The listing builds one solid part. Answer for the finished solid, in the listing's coordinates (mm). A direction names the side the tool comes from. Coordinates: 2 decimals unless noted, no trailing zeros. Loops run counter-clockwise (first coordinate to the right, second up) from the corner with the lowest first, then second, coordinate; pieces in that order, holes last. Notation, with made-up numbers: M 57.25,-38 L 69.25,-38 A27 cw 69.25,-9 Z; hole C 36.5,44.25 d2. An arc over 180 degrees is marked long. Return JSON: item names as keys, results as strings. Group by question number.
1. Given P1, Ø12, axis at y = -4.5, z = -4.5, coming from the +X side; P2, Ø5, axis at x = 4, z = 105.5, coming from the -Y side; P3, Ø7.5, axis at x = 1, z = -7.5, coming from the -Y side; P4, Ø5, axis at y = 2.5, z = 112, coming from the +X side, each flat-ended and moving along its own axis, determine where each tip first touches the part or whether it passes through.
2. The mould has two halves that part along Z. Classify faces 1 (the face through (-16, -2, 109)), 2 (the face through (2, -2, 101)), 3 (the face through (-20, 0, 59)), 4 (the face through (0, 0, -15)): pulls with the +Z half, pulls with the -Z half, needs draft (parallel to the pull), parting line crosses it, or undercut.
3. Section B-B (y = 4) is taken. Write down the section's boundary in (x, z), then the cut area to 3 significant figures.
4. Which of the six approach directions +Z, -Z, +X, -X, +Y, -Y give full straight-line access (tool end or side, diameter ignored) to faces 5 (the face through (10, 0, -7)), 6 (the face through (0, 10, -7)), 7 (the face through (2, 16, 109))?
5. Section C-C (z = -4) is taken. Write down the section's boundary in (x, y), then the cut area to 3 significant figures.
6. Section A-A (x = 14.5) is taken. Write down the section's boundary in (y, z), then the cut area to 3 significant figures.
7. Section D-D (y = -12) is taken. Write down the section's boundary in (x, z), then the cut area to 3 significant figures.
8. Straight lines are drawn through the part: L1, parallel to Z at x = -3, y = -9.5; L2, parallel to Z at x = 10.5, y = -17; L3, parallel to X at y = -8.5, z = -8. For each, find the intervals that lie inside material, in ascending order. Write a range as from..to.
```python
from build123d import *

# Parameters (mm, degrees)
F0_W     = 40
F0_H     = 40
F1_DEPTH = 120
F2_W     = 36
F2_H     = 16
F3_DEPTH = 36
F4_W     = 20
F4_H     = 20
F5_DEPTH = 15


with BuildPart() as f1:
    # F0 (on Top) → F1 (new body)
    with BuildSketch(Plane.XY):
        Rectangle(F0_W, F0_H)
    extrude(amount=F1_DEPTH)

    # F2 (on face) → F3 (cut)
    with BuildSketch(Plane.XZ.offset(20)):
        with Locations((2, 109)):
            Rectangle(F2_W, F2_H)
    extrude(amount=-F3_DEPTH, mode=Mode.SUBTRACT)

    # F4 (on face) → F5 (join)
    with BuildSketch(Plane(origin=(0, 0, 0), x_dir=(1, 0, 0), z_dir=(0, 0, -1))):
        Rectangle(F4_W, F4_H)
    extrude(amount=F5_DEPTH)


solid = f1.part
```
Worked out:
{
 "1": {"P1": "x = 20", "P2": "y = 16", "P3": "y = -10", "P4": "x = -16"},
 "2": {"face 1": "undercut", "face 2": "undercut", "face 3": "needs draft", "face 4": "pulls with the -Z half"},
 "3": {"outline": "M -20,0 L -10,0 L -10,-15 L 10,-15 L 10,0 L 20,0 L 20,101 L -16,101 L -16,117 L 20,117 L 20,120 L -20,120 Z", "area": "4,520 mm^2"},
 "4": {"face 5": "-Z, +X, +Y, -Y", "face 6": "-Z, +X, -X, +Y", "face 7": "+X, -Y"},
 "5": {"outline": "M -10,-10 L 10,-10 L 10,10 L -10,10 Z", "area": "400 mm^2"},
 "6": {"outline": "M -20,0 L 20,0 L 20,120 L -20,120 L -20,117 L 16,117 L 16,101 L -20,101 Z", "area": "4,220 mm^2"},
 "7": {"outline": "M -20,0 L 20,0 L 20,101 L -16,101 L -16,117 L 20,117 L 20,120 L -20,120 Z", "area": "4,220 mm^2"},
 "8": {"L1": "-15..101, 117..120", "L2": "0..101, 117..120", "L3": "-10..10"}
}
